Geometry: final body of the model. Coordinates: model frame, mm. A direction names the side the tool comes from. Give positions to 0.01 mm unless a question says otherwise; leave off trailing zeros. Write each loop counter-clockwise with the first axis right and the second up, starting at its lowest first coordinate (ties: lowest second). Pieces come first, ordered by that corner, then holes. Notation, with made-up numbers: (-17, 29) -> (16, 29) arc R4 cw to (16, 33) -> close; hole circle Ø1 at (33.25, 63.5). An arc over 180 degrees is marked (long way). Use CSV: the item, a comma, the result in double quotes. Start each with the question number.
1) Section D-D (x = -7.5). Output: boundary loops of the cut face in (y, z), plus the area to 3 significant figures.
2) Material intervals for line 1 (Y direction, x = 10.5, z = -38.5); line 2 (Z direction, x = 7.5, y = -12.5); line 3 (X direction, y = 22, z = -12.5), sorted ascending. Write a range as [from, to].
3) Draft query along X for faces 1 (the face through (16.002, 0, -24)), 2 (the face through (-0.42, -15.7, 2.58)), 3 (the face through (-0.42, 22.4, 2.58)), 4 (the face through (5, -23.114, -14)). Return one class per face: pulls with the +X half, pulls with the -X half, needs draft (parallel to the pull), parting line crosses it, or undercut.
4) Section A-A (x = 1.5). Output: boundary loops of the cut face in (y, z), plus the area to 3 significant figures.
5) Section C-C (z = -28). Output: boundary loops of the cut face in (x, y), plus the area to 3 significant figures.
6) Set-up query: faces 5 (the face through (5, 23.114, -14)), 6 (the face through (0, 0, 5.08)). Return all of +Z, -Z, +X, -X, +Y, -Y with unobstructed straight access to the full face (end or side cutting, diameter ignored); none if empty.
7) Contact query for flat-ended pins moving along their axis: P1, Ø6, axis at x = 0.02, y = 19.1, coming from the +Z side; P2, Ø8, axis at y = -5.5, z = -16.5, coming from the -X side; P3, Ø1, axis at x = -3, y = -11, coming from the -Z side. Output: stop coordinate, or through.
8) Section B-B (y = -13.5). Output: boundary loops of the cut face in (x, z).
```python
from build123d import *

# Parameters (mm, degrees)
SKETCH1_W           = 42.164
SKETCH1_H           = 56.388
BOSS_EXTRUDE1_DEPTH = 5.08
SKETCH2_W           = 54
SKETCH2_H           = 56.388
BOSS_EXTRUDE2_DEPTH = 5.08
SKETCH3_R           = 3.3274
CUT_EXTRUDE1_DEPTH  = 5.08
BOSS_EXTRUDE3_DEPTH = 5.08


with BuildPart() as part:
    # Sketch1 → Boss-Extrude1 (new body)
    with BuildSketch(Plane.XY):
        Rectangle(SKETCH1_W, SKETCH1_H)
    extrude(amount=BOSS_EXTRUDE1_DEPTH)

    # Sketch2 → Boss-Extrude2 (add)
    with BuildSketch(Plane(origin=(21.082, 0, 0), x_dir=(0, 0, -1), z_dir=(1, 0, 0))):
        with Locations((21.92, 0)):
            Rectangle(SKETCH2_W, SKETCH2_H)
    extrude(amount=-BOSS_EXTRUDE2_DEPTH)

    # Sketch3 → Cut-Extrude1 (cut)
    with BuildSketch(Plane.XY.offset(5.08)):
        with Locations((0.016403531, 19.102903585)):
            Circle(SKETCH3_R)
        with Locations((0.016403531, -18.997096415)):
            Circle(SKETCH3_R)
    extrude(amount=-CUT_EXTRUDE1_DEPTH, mode=Mode.SUBTRACT)

    # Sketch4 → Boss-Extrude3 (add)
    with BuildSketch(Plane(origin=(0, 28.194, 0), x_dir=(1, 0, 0), z_dir=(0, 1, 0))):
        Polygon((16.002, 48.92), (-21.082, 0), (16.002, 0), align=None)
    boss_extrude3 = extrude(amount=-BOSS_EXTRUDE3_DEPTH)

    # Mirror1: Boss-Extrude3 across plane
    add(boss_extrude3.mirror(Plane(origin=(0, 0, 0), x_dir=(0, 0, 1), z_dir=(0, -1, 0))))


solid = part.part
```
Answers follow:
1,outline,"(-28.19, -17.92) -> (-23.11, -17.92) -> (-23.11, 0) -> (23.11, 0) -> (23.11, -17.92) -> (28.19, -17.92) -> (28.19, 5.08) -> (-28.19, 5.08) -> close"
1,area,"468 mm^2"
2,line 1,"y = [-28.19, -23.11], [23.11, 28.19]"
2,line 2,"z = [0, 5.08]"
2,line 3,"x = [16, 21.08]"
3,face 1,"pulls with the -X half"
3,face 2,"undercut"
3,face 3,"undercut"
3,face 4,"needs draft"
4,outline,"(-28.19, -29.79) -> (-23.11, -29.79) -> (-23.11, 0) -> (-21.98, 0) -> (-21.98, 5.08) -> (-28.19, 5.08) -> close; (-16.02, 0) -> (16.12, 0) -> (16.12, 5.08) -> (-16.02, 5.08) -> close; (22.08, 0) -> (23.11, 0) -> (23.11, -29.79) -> (28.19, -29.79) -> (28.19, 5.08) -> (22.08, 5.08) -> close"
4,area,"529 mm^2"
5,outline,"(0.14, -28.19) -> (21.08, -28.19) -> (21.08, 28.19) -> (0.14, 28.19) -> (0.14, 23.11) -> (16, 23.11) -> (16, -23.11) -> (0.14, -23.11) -> close"
5,area,"448 mm^2"
6,face 5,"-Z, -X"
6,face 6,"+Z, +X, -X, +Y, -Y"
7,P1,"passes through"
7,P2,"stops at x = 16"
7,P3,"stops at z = 0"
8,outline,"(-21.08, 0) -> (16, 0) -> (16, -48.92) -> (21.08, -48.92) -> (21.08, 5.08) -> (-21.08, 5.08) -> close"
